```python
from build123d import *

# Parameters (mm, degrees)
SKETCH_1_R          = 1.5
EXTRUDE_1_DEPTH     = 1
SKETCH_2_R          = 2
SKETCH_2_W          = 15
SKETCH_2_H          = 20
CUT_EXTRUDE_1_DEPTH = 315.198981539
CUT_EXTRUDE_2_REACH = 316.199
FILLET_1_R          = 3


with BuildPart() as part:
    # 草图1 → 凸台-拉伸1 (new body)
    with BuildSketch(Plane.XY):
        Polygon((0, 0), (0, 76), (25, 76), (25, 116), (267, 116), (267, 76), (292, 76), (292, 0), align=None)
        with Locations((3, 48)):
            Circle(SKETCH_1_R, mode=Mode.SUBTRACT)
        with Locations((3, 28)):
            Circle(SKETCH_1_R, mode=Mode.SUBTRACT)
        with Locations(Location((289, 28, 0), (0, 0, 180))):
            Circle(SKETCH_1_R, mode=Mode.SUBTRACT)
        with Locations(Location((289, 48, 0), (0, 0, 180))):
            Circle(SKETCH_1_R, mode=Mode.SUBTRACT)
    extrude(amount=EXTRUDE_1_DEPTH)

    # 草图2 → 切除-拉伸1 (cut, through all)
    with BuildSketch(Plane.XY.offset(1)):
        with Locations((65, 111)):
            Circle(SKETCH_2_R)
        with Locations(Location((227, 111, 0), (0, 0, 180))):
            Circle(SKETCH_2_R)
        with Locations((146, 111)):
            Circle(SKETCH_2_R)
        with Locations((193.5, 106)):
            Rectangle(SKETCH_2_W, SKETCH_2_H)
        with Locations((98.5, 106)):
            Rectangle(SKETCH_2_W, SKETCH_2_H)
    extrude(amount=-CUT_EXTRUDE_1_DEPTH, mode=Mode.SUBTRACT)

    # 草图3 → 切除-拉伸2 (cut, up to next)
    with BuildSketch(Plane(origin=(0, 0, 0), x_dir=(-1, 0, 0), z_dir=(0, 0, -1)), mode=Mode.PRIVATE) as cut_extrude_2_sk1:
        Polygon((-43.02940934, 35.888888889), (-78.02940934, 81), (-43.02940934, 81), align=None)
    cut_extrude_2_tool1 = extrude(cut_extrude_2_sk1.sketch, amount=-CUT_EXTRUDE_2_REACH, mode=Mode.PRIVATE) & part.part
    # 草图3 → 切除-拉伸2 (cut, up to next)
    with BuildSketch(Plane(origin=(0, 0, 0), x_dir=(-1, 0, 0), z_dir=(0, 0, -1)), mode=Mode.PRIVATE) as cut_extrude_2_sk2:
        Polygon((-127.01470467, 23), (-52.01470467, 23), (-89.51470467, 71.333333333), align=None)
    cut_extrude_2_tool2 = extrude(cut_extrude_2_sk2.sketch, amount=-CUT_EXTRUDE_2_REACH, mode=Mode.PRIVATE) & part.part
    # 草图3 → 切除-拉伸2 (cut, up to next)
    with BuildSketch(Plane(origin=(0, 0, 0), x_dir=(-1, 0, 0), z_dir=(0, 0, -1)), mode=Mode.PRIVATE) as cut_extrude_2_sk3:
        Polygon((-101, 81), (-146, 81), (-146, 23), align=None)
    cut_extrude_2_tool3 = extrude(cut_extrude_2_sk3.sketch, amount=-CUT_EXTRUDE_2_REACH, mode=Mode.PRIVATE) & part.part
    # 草图3 → 切除-拉伸2 (cut, up to next)
    with BuildSketch(Plane(origin=(0, 0, 0), x_dir=(-1, 0, 0), z_dir=(0, 0, -1)), mode=Mode.PRIVATE) as cut_extrude_2_sk4:
        Polygon((-202.48529533, 71.333333333), (-164.98529533, 23), (-239.98529533, 23), align=None)
    cut_extrude_2_tool4 = extrude(cut_extrude_2_sk4.sketch, amount=-CUT_EXTRUDE_2_REACH, mode=Mode.PRIVATE) & part.part
    # 草图3 → 切除-拉伸2 (cut, up to next)
    with BuildSketch(Plane(origin=(0, 0, 0), x_dir=(-1, 0, 0), z_dir=(0, 0, -1)), mode=Mode.PRIVATE) as cut_extrude_2_sk5:
        Polygon((-146, 81), (-191, 81), (-146, 23), align=None)
    cut_extrude_2_tool5 = extrude(cut_extrude_2_sk5.sketch, amount=-CUT_EXTRUDE_2_REACH, mode=Mode.PRIVATE) & part.part
    # 草图3 → 切除-拉伸2 (cut, up to next)
    with BuildSketch(Plane(origin=(0, 0, 0), x_dir=(-1, 0, 0), z_dir=(0, 0, -1)), mode=Mode.PRIVATE) as cut_extrude_2_sk6:
        Polygon((-248.97059066, 35.888888889), (-213.97059066, 81), (-248.97059066, 81), align=None)
    cut_extrude_2_tool6 = extrude(cut_extrude_2_sk6.sketch, amount=-CUT_EXTRUDE_2_REACH, mode=Mode.PRIVATE) & part.part
    add(cut_extrude_2_tool1.solids().sort_by_distance((54.696076, 65.962963, 0))[0], mode=Mode.SUBTRACT)
    add(cut_extrude_2_tool2.solids().sort_by_distance((89.514705, 39.111111, 0))[0], mode=Mode.SUBTRACT)
    add(cut_extrude_2_tool3.solids().sort_by_distance((131, 61.666667, 0))[0], mode=Mode.SUBTRACT)
    add(cut_extrude_2_tool4.solids().sort_by_distance((202.485295, 39.111111, 0))[0], mode=Mode.SUBTRACT)
    add(cut_extrude_2_tool5.solids().sort_by_distance((161, 61.666667, 0))[0], mode=Mode.SUBTRACT)
    add(cut_extrude_2_tool6.solids().sort_by_distance((237.303924, 65.962963, 0))[0], mode=Mode.SUBTRACT)

    # 圆角1
    fillet_1_edges = [part.edges().sort_by_distance(p)[0] for p in [
        (52.01470467, 23, 0.5),
        (127.01470467, 23, 0.5),
        (89.51470467, 71.333333333, 0.5),
        (202.48529533, 71.333333333, 0.5),
        (164.98529533, 23, 0.5),
        (239.98529533, 23, 0.5),
        (191, 81, 0.5),
        (101, 81, 0.5),
        (146, 23, 0.5),
        (213.97059066, 81, 0.5),
        (248.97059066, 35.888888889, 0.5),
        (248.97059066, 81, 0.5),
        (43.02940934, 35.888888889, 0.5),
        (78.02940934, 81, 0.5),
        (43.02940934, 81, 0.5),
    ]]
    fillet(fillet_1_edges, radius=FILLET_1_R)


solid = part.part
```
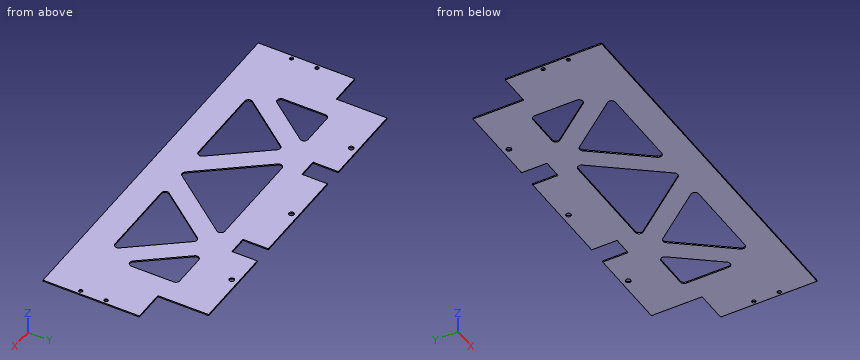
Input: part model. Units: mm. Frame: model coordinates. Coordinates: 2 decimals unless noted, no trailing zeros. Loops run counter-clockwise (first coordinate to the right, second up) from the corner with the lowest first, then second, coordinate; pieces in that order, holes last. Notation, with made-up numbers: (-9, -16) - (30, -16) arc R29 ccw to (30, 6) - close; hole circle Ø9 at (84, 57.5). An arc over 180 degrees is marked (long way). Answer in a Markdown table with one row per item.
(1) Material intervals for L1, parallel to Y at x = 3, z = 0.8; L2, parallel to Y at x = 171.5, z = 0.9; L3, parallel to Y at x = 203, z = 0.8, sorted ascending. Write a range as from..to.
Model answer:
| item | result |
|---|---|
| L1 | y = 0..26.5, 29.5..46.5, 49.5..76 |
| L2 | y = 0..23, 31.4..55.87, 81..116 |
| L3 | y = 0..23, 69.39..116 |
(2) Cut plane A-A on y = 103. Output: boundary loops of the cut face in (x, z), plus the area to 3 significant figures.
Model answer:
| item | result |
|---|---|
| outline | (25, 0) - (91, 0) - (91, 1) - (25, 1) - close; (106, 0) - (186, 0) - (186, 1) - (106, 1) - close; (201, 0) - (267, 0) - (267, 1) - (201, 1) - close |
| area | 212 mm² |
(3) Cut plane C-C on x = 99. Output: boundary loops of the cut face in (y, z).
Model answer:
| item | result |
|---|---|
| outline | (0, 0) - (23, 0) - (23, 1) - (0, 1) - close; (59.11, 0) - (96, 0) - (96, 1) - (59.11, 1) - close |
(4) Pin query (flat end, axial travel): P1, Ø0.5, axis at x = 96, z = 0.5, coming from the +Y side. Return the tip coordinate at first contact, or that it passes through.
Model answer:
| item | result |
|---|---|
| P1 | stops at y = 96 |
(5) Cut plane D-D on z = 0.85. Count the separate pieces of the cut face and the enclosed holes in it, plus the area to 3 significant figures.
Model answer:
| item | result |
|---|---|
| separate pieces | 1 |
| enclosed holes | 12 |
| area | 23,500 mm² |
(6) Cut plane B-B on y = 72. Output: boundary loops of the cut face in (x, z).
Model answer:
| item | result |
|---|---|
| outline | (0, 0) - (43.03, 0) - (43.03, 1) - (0, 1) - close; (71.05, 0) - (107.98, 0) - (107.98, 1) - (71.05, 1) - close; (184.02, 0) - (220.95, 0) - (220.95, 1) - (184.02, 1) - close; (248.97, 0) - (292, 0) - (292, 1) - (248.97, 1) - close |
